```python
from build123d import *

# Parameters (mm, degrees)
SALIENTE_EXTRUIR1_DEPTH = 45
CROQUIS3_R              = 6
CORTAR_EXTRUIR1_DEPTH   = 61
CROQUIS3_4_R            = 12
CROQUIS3_4_R_2          = 6
CORTAR_EXTRUIR2_DEPTH   = 9
CROQUIS4_R              = 12
CORTAR_EXTRUIR3_DEPTH   = 9
SALIENTE_EXTRUIR3_DEPTH = 45
CORTAR_EXTRUIR4_DEPTH   = 18
CORTAR_EXTRUIR5_DEPTH   = 18
SALIENTE_EXTRUIR4_DEPTH = 45
CROQUIS8_R              = 6
CORTAR_EXTRUIR7_DEPTH   = 61
CROQUIS9_R              = 12
CORTAR_EXTRUIR8_DEPTH   = 9
CROQUIS10_R             = 12
CORTAR_EXTRUIR9_DEPTH   = 9
SALIENTE_EXTRUIR7_DEPTH = 60
CORTAR_EXTRUIR10_DEPTH  = 52.977922061
CORTAR_EXTRUIR11_DEPTH  = 52.977922061
CROQUIS21_R             = 7.5
CORTAR_EXTRUIR13_DEPTH  = 52.977922061


with BuildPart() as part:
    # Croquis2 → Saliente-Extruir1 (new body)
    with BuildSketch(Plane(origin=(0, 0, 0), x_dir=(1, 0, 0), z_dir=(0, 1, 0))):
        with BuildLine():
            Line((-12, 9), (-60, 9))
            Line((-60, 9), (-60, 30))
            Line((-60, 30), (0, 30))
            ThreePointArc((0, 30), (30, 0), (0, -30))
            Line((0, -30), (-60, -30))
            Line((-60, -30), (-60, -9))
            Line((-60, -9), (-12, -9))
            ThreePointArc((-12, -9), (15, 0), (-12, 9))
        make_face()
    extrude(amount=SALIENTE_EXTRUIR1_DEPTH)

    # Croquis3 → Cortar-Extruir1 (cut, through all)
    with BuildSketch(Plane.XY.offset(30)):
        with Locations((-36, 22.5)):
            Circle(CROQUIS3_R)
    extrude(amount=-CORTAR_EXTRUIR1_DEPTH, mode=Mode.SUBTRACT)

    # Croquis3_4 → Cortar-Extruir2 (cut)
    with BuildSketch(Plane.XY.offset(30)):
        with Locations((-36, 22.5)):
            Circle(CROQUIS3_4_R)
        with Locations((-36, 22.5)):
            Circle(CROQUIS3_4_R_2, mode=Mode.SUBTRACT)
    extrude(amount=-CORTAR_EXTRUIR2_DEPTH, mode=Mode.SUBTRACT)

    # Croquis4 → Cortar-Extruir3 (cut)
    with BuildSketch(Plane(origin=(0, 0, -30), x_dir=(-1, 0, 0), z_dir=(0, 0, -1))):
        with Locations((36, 22.5)):
            Circle(CROQUIS4_R)
    extrude(amount=-CORTAR_EXTRUIR3_DEPTH, mode=Mode.SUBTRACT)

    # Croquis5 → Saliente-Extruir3 (add, through all)
    with BuildSketch(Plane(origin=(0, 45, 0), x_dir=(1, 0, 0), z_dir=(0, 1, 0))):
        with BuildLine():
            Line((51, 0), (51, -30))
            Line((51, -30), (0, -30))
            ThreePointArc((0, -30), (30, 0), (0, 30))
            Line((0, 30), (90, 30))
            Line((90, 30), (90, -30))
            Line((90, -30), (69, -30))
            Line((69, -30), (69, 0))
            ThreePointArc((69, 0), (60, 9), (51, 0))
        make_face()
    extrude(amount=-SALIENTE_EXTRUIR3_DEPTH)

    # Croquis6 → Cortar-Extruir4 (cut)
    with BuildSketch(Plane(origin=(0, 45, 0), x_dir=(1, 0, 0), z_dir=(0, 1, 0))):
        with BuildLine():
            Line((69, -30), (90, -30))
            Line((90, -30), (90, 30))
            Line((90, 30), (0, 30))
            Line((0, 30), (0, 15))
            ThreePointArc((0, 15), (15, 0), (0, -15))
            Line((0, -15), (0, -30))
            Line((0, -30), (51, -30))
            Line((51, -30), (51, 0))
            ThreePointArc((51, 0), (60, 9), (69, 0))
            Line((69, 0), (69, -30))
        make_face()
    extrude(amount=-CORTAR_EXTRUIR4_DEPTH, mode=Mode.SUBTRACT)

    # Croquis7 → Cortar-Extruir5 (cut)
    with BuildSketch(Plane.XZ):
        with BuildLine():
            Line((51, 30), (51, 0))
            ThreePointArc((51, 0), (60, -9), (69, 0))
            Line((69, 0), (69, 30))
            Line((69, 30), (90, 30))
            Line((90, 30), (90, -30))
            Line((90, -30), (0, -30))
            Line((0, -30), (0, -15))
            ThreePointArc((0, -15), (15, 0), (0, 15))
            Line((0, 15), (0, 30))
            Line((0, 30), (51, 30))
        make_face()
    extrude(amount=-CORTAR_EXTRUIR5_DEPTH, mode=Mode.SUBTRACT)

    # Croquis2_3 → Saliente-Extruir4 (add)
    with BuildSketch(Plane(origin=(0, 0, 0), x_dir=(1, 0, 0), z_dir=(0, 1, 0))):
        with BuildLine():
            Line((-12, 9), (-60, 9))
            Line((-60, 9), (-60, 30))
            Line((-60, 30), (0, 30))
            ThreePointArc((0, 30), (30, 0), (0, -30))
            Line((0, -30), (-60, -30))
            Line((-60, -30), (-60, -9))
            Line((-60, -9), (-12, -9))
            ThreePointArc((-12, -9), (15, 0), (-12, 9))
        make_face()
    extrude(amount=SALIENTE_EXTRUIR4_DEPTH)

    # Croquis8 → Cortar-Extruir7 (cut, through all)
    with BuildSketch(Plane.XY.offset(30)):
        with Locations((-36, 22.5)):
            Circle(CROQUIS8_R)
    extrude(amount=-CORTAR_EXTRUIR7_DEPTH, mode=Mode.SUBTRACT)

    # Croquis9 → Cortar-Extruir8 (cut)
    with BuildSketch(Plane.XY.offset(30)):
        with Locations((-36, 22.5)):
            Circle(CROQUIS9_R)
    extrude(amount=-CORTAR_EXTRUIR8_DEPTH, mode=Mode.SUBTRACT)

    # Croquis10 → Cortar-Extruir9 (cut)
    with BuildSketch(Plane(origin=(0, 0, -30), x_dir=(-1, 0, 0), z_dir=(0, 0, -1))):
        with Locations((36, 22.5)):
            Circle(CROQUIS10_R)
    extrude(amount=-CORTAR_EXTRUIR9_DEPTH, mode=Mode.SUBTRACT)

    # Croquis16 → Saliente-Extruir7 (add, through all)
    with BuildSketch(Plane.XY.offset(30)):
        Polygon((90, 18), (132.779960262, 60.779960262), (126.415999231, 67.143921292), (83.636038969, 24.363961031), align=None)
    extrude(amount=-SALIENTE_EXTRUIR7_DEPTH)

    # Croquis18 → Cortar-Extruir10 (cut, through all)
    with BuildSketch(Plane(origin=(29.636038969, -29.636038969, 0), x_dir=(0, 0, 1), z_dir=(-0.707106781, 0.707106781, 0))):
        with BuildLine():
            Line((-30, 136.867532368), (-30, 80.09545443))
            Line((-30, 80.09545443), (-14.205841491, 126.68355433))
            ThreePointArc((-14.205841491, 126.68355433), (-8.739555783, 134.058519396), (0, 136.867532368))
            Line((0, 136.867532368), (-30, 136.867532368))
        make_face()
    extrude(amount=-CORTAR_EXTRUIR10_DEPTH, mode=Mode.SUBTRACT)

    # Croquis19 → Cortar-Extruir11 (cut, through all)
    with BuildSketch(Plane(origin=(29.636038969, -29.636038969, 0), x_dir=(0, 0, 1), z_dir=(-0.707106781, 0.707106781, 0))):
        with BuildLine():
            Line((30, 80.09545443), (14.205841491, 126.68355433))
            ThreePointArc((14.205841491, 126.68355433), (8.739555783, 134.058519396), (0, 136.867532368))
            Line((0, 136.867532368), (30, 136.867532368))
            Line((30, 136.867532368), (30, 80.09545443))
        make_face()
    extrude(amount=-CORTAR_EXTRUIR11_DEPTH, mode=Mode.SUBTRACT)

    # Croquis21 → Cortar-Extruir13 (cut, through all)
    with BuildSketch(Plane(origin=(29.636038969, -29.636038969, 0), x_dir=(0, 0, 1), z_dir=(-0.707106781, 0.707106781, 0))):
        with Locations((0, 121.867532368)):
            Circle(CROQUIS21_R)
    extrude(amount=-CORTAR_EXTRUIR13_DEPTH, mode=Mode.SUBTRACT)


solid = part.part
```
Model file for the job. Use its own axes, mm. A direction names the side the tool comes from. Give positions to 0.01 mm unless a question says otherwise; leave off trailing zeros. Write each loop counter-clockwise with the first axis right and the second up, starting at its lowest first coordinate (ties: lowest second). Pieces come first, ordered by that corner, then holes. Notation, with made-up numbers: M -21.75,50 L 19.25,50 A12 ccw 19.25,58 Z; hole C 45,41 d2. An arc over 180 degrees is marked long. Use a Markdown table: item, result.
1) Cut at A-A (x = -36). List the corners of the cut face in (y, z).
Responses:
| item | result |
|---|---|
| outline | M 0,-30 L 10.5,-30 L 10.5,-21 L 16.5,-21 L 16.5,-9 L 0,-9 Z; M 0,9 L 16.5,9 L 16.5,21 L 10.5,21 L 10.5,30 L 0,30 Z; M 28.5,-21 L 34.5,-21 L 34.5,-30 L 45,-30 L 45,-9 L 28.5,-9 Z; M 28.5,9 L 45,9 L 45,30 L 34.5,30 L 34.5,21 L 28.5,21 Z |
2) Drill centre lines: line 1 (Z direction, x = -26.5, y = 12.5); line 2 (Y direction, x = -36, z = 12); line 3 (Z direction, x = 0, y = 21). Where is each one in solid material? Low to high. Write a range as from..to.
Responses:
| item | result |
|---|---|
| line 1 | z = -30..-9, 9..30 |
| line 2 | y = 0..16.5, 28.5..45 |
| line 3 | z = -30..-15, 15..30 |
3) Pull direction Y, two halves, no side cores. Call faces 1 (the cylindrical face through (-41.994, 22.764, 15.084)), 2 (the flat face through (69, 23, 15)), 3 (the flat face through (46, 18, 0)): +Y half, -Y half, draft (parallel to the pull), parting line (faces both ways), or undercut.
Responses:
| item | result |
|---|---|
| face 1 | undercut |
| face 2 | draft |
| face 3 | -Y half |
4) Pin check, flat tips, straight feed: pin 1 (21.5 mm diameter, centred on x = -36, y = 22.5, fed in from +Z); pin 2 (18 mm diameter, centred on x = 66, z = 8.5, fed in from -Y); pin 3 (4.5 mm diameter, centred on y = 23, z = 17, fed in from +X); pin 4 (9.5 mm diameter, centred on x = -36, y = 22.5, fed in from +Z). Stop position of each tip, or through.
Responses:
| item | result |
|---|---|
| pin 1 | stops at z = 21 |
| pin 2 | stops at y = 18 |
| pin 3 | stops at x = 97.25 |
| pin 4 | passes through |
5) Cut at B-B (z = 24). List the corners of the cut face in (x, y), and give its area (3 significant figures).
Responses:
| item | result |
|---|---|
| outline | M -60,0 L 18,0 L 18,18 L 51,18 L 51,27 L 18,27 L 18,45 L -60,45 Z; M 69,18 L 90,18 L 105.15,33.15 L 98.79,39.51 L 86.27,27 L 69,27 Z; hole C -36,22.5 d24 |
| area | 3,700 mm2 |
6) Cut at C-C (y = 22.5). Give the number of separate pieces and of enclosed holes in the cut face, and give its area (3 significant figures).
Responses:
| item | result |
|---|---|
| separate pieces | 3 |
| enclosed holes | 0 |
| area | 6,350 mm2 |
7) Cut at D-D (x = 2.5). List the corners of the cut face in (y, z), and give its area (3 significant figures).
Responses:
| item | result |
|---|---|
| outline | M 0,-29.9 L 18,-29.9 L 18,-30 L 27,-30 L 27,-29.9 L 45,-29.9 L 45,-14.79 L 0,-14.79 Z; M 0,14.79 L 45,14.79 L 45,29.9 L 27,29.9 L 27,30 L 18,30 L 18,29.9 L 0,29.9 Z |
| area | 1,360 mm2 |
8) Tool access for faces 4 (the flat face through (-14, 45, -14)), 5 (the flat face through (-30, 20, -21)), 6 (the flat face through (102.16, 42.89, 0.42)), 7 (the flat face through (-30, 17, -9)): list every direction of +Z, -Z, +X, -X, +Y, -Y with a clear straight run to the whole face (end or side of a thin tool).
Responses:
| item | result |
|---|---|
| face 4 | +Z, -Z, -X, +Y |
| face 5 | -Z |
| face 6 | +Z, -Z, +Y |
| face 7 | -X, +Y, -Y |
